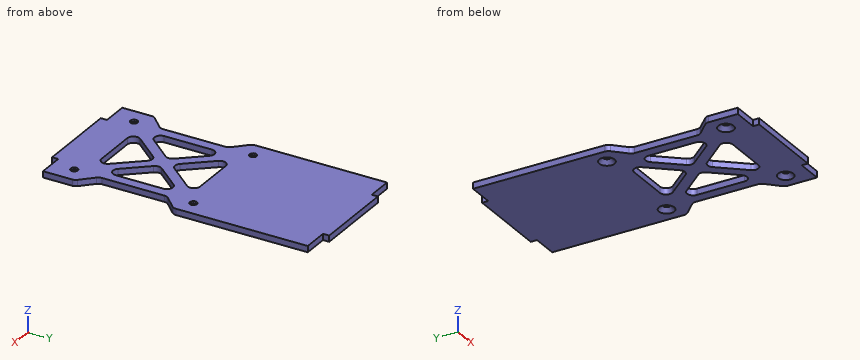
```python
from build123d import *

# Parameters (mm, degrees)
SKETCH_1_W          = 65
SKETCH_1_H          = 129
SKETCH_1_W_2        = 40
SKETCH_1_H_2        = 6
EXTRUDE_1_DEPTH     = 3
SKETCH_2_R          = 1.75
CUT_EXTRUDE_1_DEPTH = 10
CHAMFER_1_SIZE      = 2
CUT_EXTRUDE_2_DEPTH = 10
FILLET_1_R          = 3
FILLET_2_R          = 3
FILLET_3_R          = 3


with BuildPart() as part:
    # Эскиз1 → Бобышка-Вытянуть1 (new body)
    with BuildSketch(Plane.XY):
        Rectangle(SKETCH_1_W, SKETCH_1_H)
        with Locations((0, 64.5)):
            Rectangle(SKETCH_1_W_2, SKETCH_1_H_2)
        with Locations((0, -64.5)):
            Rectangle(SKETCH_1_W_2, SKETCH_1_H_2)
    extrude(amount=EXTRUDE_1_DEPTH)

    # Эскиз2 → Вырез-Вытянуть1 (cut)
    with BuildSketch(Plane.XY.offset(3)):
        with Locations((-24.5, 4)):
            Circle(SKETCH_2_R)
        with Locations((24.5, 4)):
            Circle(SKETCH_2_R)
        with Locations((24.5, -54)):
            Circle(SKETCH_2_R)
        with Locations((-24.5, -54)):
            Circle(SKETCH_2_R)
    extrude(amount=-CUT_EXTRUDE_1_DEPTH, mode=Mode.SUBTRACT)

    # Фаска1
    chamfer_1_edges = [part.edges().sort_by_distance(p)[0] for p in [
        (-26.25, -54, 0),
        (22.75, -54, 0),
        (22.75, 4, 0),
        (-26.25, 4, 0),
    ]]
    chamfer(chamfer_1_edges, length=CHAMFER_1_SIZE)

    # Эскиз3 → Вырез-Вытянуть2 (cut)
    with BuildSketch(Plane(origin=(0, 0, 0), x_dir=(-1, 0, 0), z_dir=(0, 0, -1))):
        Polygon((32.5, -1), (25, -8.5), (25, -41.5), (32.5, -49), (35.92761887, -49), (35.92761887, -1), align=None)
        Polygon((-35.92761887, -49), (-32.5, -49), (-25, -41.5), (-25, -8.5), (-32.5, -1), (-35.92761887, -1), align=None)
        Polygon((0, -21.126143006), (-17.003120815, -1), (17.003120815, -1), align=None)
        Polygon((20, -5.200387607), (3.272741254, -25), (20, -44.799612393), align=None)
        Polygon((17.003120815, -49), (0, -28.873856994), (-17.003120815, -49), align=None)
        Polygon((-20, -5.200387607), (-20, -44.799612393), (-3.272741254, -25), align=None)
    extrude(amount=-CUT_EXTRUDE_2_DEPTH, mode=Mode.SUBTRACT)

    # Скругление1
    fillet_1_edges = [part.edges().sort_by_distance(p)[0] for p in [
        (-32.5, -1, 1.5),
        (-32.5, -49, 1.5),
        (-25, -41.5, 1.5),
        (-25, -8.5, 1.5),
    ]]
    fillet(fillet_1_edges, radius=FILLET_1_R)

    # Скругление2
    fillet_2_edges = [part.edges().sort_by_distance(p)[0] for p in [
        (32.5, -1, 1.5),
        (25, -8.5, 1.5),
        (25, -41.5, 1.5),
        (32.5, -49, 1.5),
    ]]
    fillet(fillet_2_edges, radius=FILLET_2_R)

    # Скругление3
    fillet_3_edges = [part.edges().sort_by_distance(p)[0] for p in [
        (17.003120815, -49, 1.5),
        (0, -28.873856994, 1.5),
        (-17.003120815, -49, 1.5),
        (-20, -44.799612393, 1.5),
        (-3.272741254, -25, 1.5),
        (-20, -5.200387607, 1.5),
        (3.272741254, -25, 1.5),
        (20, -44.799612393, 1.5),
        (20, -5.200387607, 1.5),
        (-17.003120815, -1, 1.5),
        (0, -21.126143006, 1.5),
        (17.003120815, -1, 1.5),
    ]]
    fillet(fillet_3_edges, radius=FILLET_3_R)


solid = part.part
```
Work out the finished part from the listing and answer in its coordinate system (mm). Give positions to 0.01 mm unless a question says otherwise; leave off trailing zeros. Loops run counter-clockwise (first coordinate to the right, second up) from the corner with the lowest first, then second, coordinate; pieces in that order, holes last. Notation, with made-up numbers: (54.5, -8.75) -> (80.5, -8.75) arc R27 cw to (80.5, 27.25) -> close; hole circle Ø9 at (-2, 83.25). An arc over 180 degrees is marked (long way). Write item = value, one per line. Start each with the question number.
(1) Find section B-B on z = 0.8. Give the number of separate pieces and of enclosed holes in the cut face, and give its area (3 significant figures).
(2) Find the intervals of material crossed by probe 1 along Y at (x, z) = (-24.5, 2.8); probe 2 along X at (y, z) = (-23, 2); probe 3 along X at (y, z) = (-27.5, 1.5), in increasing order. Write a range as from..to.
(3) Find section A-A on y = -54. Give the vertices of the cut face in (x, z), and give its area (3 significant figures).
(4) Given pin 1 Ø0.9 at (y, z) = (-17.5, 1) entering from +X; pin 2 Ø1.5 at (y, z) = (66.5, 2) entering from +X; pin 3 Ø1.5 at (x, z) = (-23.5, 2) entering from +Y; pin 4 Ø3 at (x, y) = (24.5, -54) entering from -Z, each flat-ended and moving along its own axis, determine where each tip first touches the part or whether it passes through.
From the geometry:
q1.separate_pieces = 1
q1.enclosed_holes = 8
q1.area = 6,660 mm^2
q2.probe_1 = -64.5..-55.75, -52.25..2.25, 5.75..64.5
q2.probe_2 = -25..-20, -4.96..4.96, 20..25
q2.probe_3 = -25..-20, -5.38..5.38, 20..25
q3.outline = (-32.5, 0) -> (-28.25, 0) -> (-26.25, 2) -> (-26.25, 3) -> (-32.5, 3) -> close; (-22.75, 2) -> (-20.75, 0) -> (20.75, 0) -> (22.75, 2) -> (22.75, 3) -> (-22.75, 3) -> close; (26.25, 2) -> (28.25, 0) -> (32.5, 0) -> (32.5, 3) -> (26.25, 3) -> close
q3.area = 166 mm^2
q4.pin_1 = 25
q4.pin_2 = 20
q4.pin_3 = 64.5
q4.pin_4 = through
